The listing builds one solid part. Answer for the finished solid, in the listing's coordinates (mm). Coordinates: 2 decimals unless noted, no trailing zeros. Write each loop counter-clockwise with the first axis right and the second up, starting at its lowest first coordinate (ties: lowest second). Pieces come first, ordered by that corner, then holes.
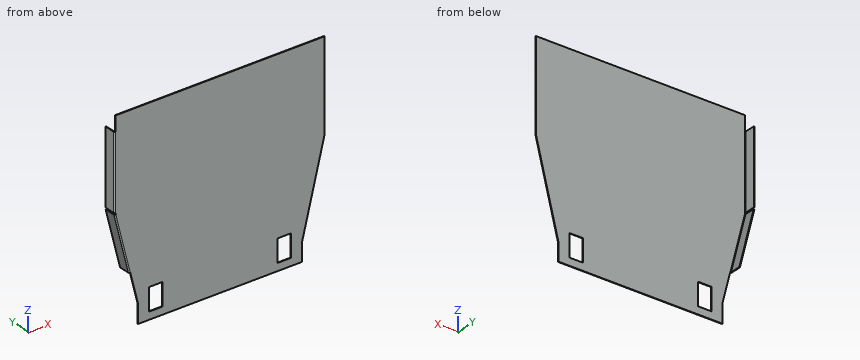
```python
from build123d import *

# Parameters (mm, degrees)
SKETCH7_W          = 280
SKETCH7_H          = 120
BASE_FLANGE4_DEPTH = 0.8
TAB2_DEPTH         = 0.8
SKETCH11_W         = 18
SKETCH11_H         = 30
CUT_EXTRUDE1_DEPTH = 249.245120798
EDGE_FLANGE1_DEPTH = 99
EDGE_FLANGE2_DEPTH = 80


# Sheet-metal steps are written as plain solids
with BuildPart() as part:
    # Sketch7 → Base-Flange4 (new body)
    with BuildSketch(Plane(origin=(0, 0, 0), x_dir=(1, 0, 0), z_dir=(0, 1, 0))):
        Rectangle(SKETCH7_W, SKETCH7_H)
    extrude(amount=-BASE_FLANGE4_DEPTH)

    # Sketch10 → Tab2 (add)
    with BuildSketch(Plane(origin=(0, 0, 0), x_dir=(1, 0, 0), z_dir=(0, 1, 0))):
        Polygon((140, 60), (-140, 60), (-110, 180), (-110, 205), (110, 205), (110, 180), align=None)
    extrude(amount=-TAB2_DEPTH)

    # Sketch11 → Cut-Extrude1 (cut, through all)
    with BuildSketch(Plane(origin=(0, 0, 0), x_dir=(1, 0, 0), z_dir=(0, 1, 0))):
        with Locations((-86, 180)):
            Rectangle(SKETCH11_W, SKETCH11_H)
        with Locations((86, 180)):
            Rectangle(SKETCH11_W, SKETCH11_H)
    extrude(amount=-CUT_EXTRUDE1_DEPTH, mode=Mode.SUBTRACT)

    # Edge-Flange1 section (across the edge) → Edge-Flange1 (add)
    with BuildSketch(Plane(origin=(-140.7366, 0, -59), x_dir=(1, 0, 0), z_dir=(0, 0, 1))):
        with BuildLine():
            Line((-0.8, 0.7366), (-0.8, 15))
            Line((-0.8, 15), (0, 15))
            Line((0, 15), (0, 0.7366))
            ThreePointArc((0, 0.7366), (0.215745145, 0.215745145), (0.7366, 0))
            Line((0.7366, 0), (0.7366, -0.8))
            ThreePointArc((0.7366, -0.8), (-0.34994028, -0.34994028), (-0.8, 0.7366))
        make_face()
    extrude(amount=EDGE_FLANGE1_DEPTH)

    # Edge-Flange2 section (across the edge) → Edge-Flange2 (add)
    with BuildSketch(Plane(origin=(-121.069221338, 0, -138.760194253), x_dir=(0.9701425001453319, 3.4914813388431334e-15, 0.24253562503633339), z_dir=(-0.24253562503633339, 0, 0.9701425001453319))):
        with BuildLine():
            Line((-0.8, 0.7366), (-0.8, 15))
            Line((-0.8, 15), (0, 15))
            Line((0, 15), (0, 0.7366))
            ThreePointArc((0, 0.7366), (0.215745145, 0.215745145), (0.7366, 0))
            Line((0.7366, 0), (0.7366, -0.8))
            ThreePointArc((0.7366, -0.8), (-0.34994028, -0.34994028), (-0.8, 0.7366))
        make_face()
    extrude(amount=EDGE_FLANGE2_DEPTH)


solid = part.part
```
(1) Section A-A, the plane y = 10 is taken. Write down the section's boundary in (x, z).
(2) Section C-C, the plane x = 70 is taken. Write down the section's boundary in (y, z).
(3) Section B-B, the plane z = -30.5 is taken. Write down the section's boundary in (x, y).
(4) Each of these flat-tipped pins is pushed along its axis until it touches: pin 1 (3 mm diameter, centred on x = -82, z = -144.5, fed in from +Y); pin 2 (0.6 mm diameter, centred on y = -0.5, z = -180.5, fed in from -X); pin 3 (0.9 mm diameter, centred on y = -0.5, z = -59.5, fed in from -X). Where does it stop, or does it pass through?
(5) Find the intervals of material crossed by probe 1 along Y at (x, z) = (-96.5, 19.5); probe 2 along X at (y, z) = (3, 5); probe 3 along X at (y, z) = (3, -120), in increasing order.
Solution:
1. outline: (-141.54, -59) - (-140.74, -59) - (-140.74, 40) - (-141.54, 40) - close; (-141.25, -61.34) - (-121.85, -138.95) - (-121.07, -138.76) - (-140.47, -61.15) - close
2. outline: (-0.8, -205) - (0, -205) - (0, 60) - (-0.8, 60) - close
3. outline: (-141.54, 0.74) arc R1.54 ccw to (-140, -0.8) - (140, -0.8) - (140, 0) - (-140, 0) arc R0.74 cw to (-140.74, 0.74) - (-140.74, 15) - (-141.54, 15) - close
4. pin 1: stops at y = 0
4. pin 2: stops at x = -110
4. pin 3: stops at x = -140
5. probe 1: y = -0.8 to 0
5. probe 2: x = -141.54 to -140.74
5. probe 3: x = -126.58 to -125.76
